```python
from build123d import *

# Parameters (mm, degrees)
F1_DEPTH = 2.794
F2_R     = 23.5
F3_DEPTH = 15
F5_D     = 12.1
F7_D     = 9
F7_DEPTH = 3
F7_TIP   = 2.7038727856
F9_D     = 17
F9_DEPTH = 2
F9_TIP   = 5.1073152617


with BuildPart() as f1:
    # F0 (on Front) → F1 (new body)
    with BuildSketch(Plane.XZ):
        Polygon((-22.3028203132, 16.203947452), (-27.5678019971, 0), (-22.3028203132, -16.203947452), (-8.5189193147, -26.2185377292), (8.5189193147, -26.2185377292), (22.3028203132, -16.203947452), (27.5678019971, 0), (22.3028203132, 16.203947452), (8.5189193147, 26.2185377292), (-8.5189193147, 26.2185377292), align=None)
    extrude(amount=F1_DEPTH)

    # F2 (on face) → F3 (join)
    with BuildSketch(Plane.XZ.offset(2.794)):
        Circle(F2_R)
    extrude(amount=F3_DEPTH)

    # F5 (through all)
    with Locations(Plane.XZ.offset(17.794)):
        with Locations((-14, 0), (0, 14), (14, 0), (0, -14)):
            Hole(F5_D / 2)

    # F7
    with Locations(Plane(origin=(0, 0, 0), x_dir=(-1, 0, 0), z_dir=(0, 1, 0))):
        with Locations((0, 0)):
            Hole(F7_D / 2, depth=F7_DEPTH)
            with Locations((0, 0, -(F7_DEPTH + F7_TIP / 2))):  # 118° drill point
                Cone(0, F7_D / 2, F7_TIP, mode=Mode.SUBTRACT)

    # F9
    with Locations(Plane(origin=(0, 0, 0), x_dir=(-1, 0, 0), z_dir=(0, 1, 0))):
        with Locations((-14, 0), (0, 14), (14, 0), (0, -14)):
            Hole(F9_D / 2, depth=F9_DEPTH)
            with Locations((0, 0, -(F9_DEPTH + F9_TIP / 2))):  # 118° drill point
                Cone(0, F9_D / 2, F9_TIP, mode=Mode.SUBTRACT)


solid = f1.part
```
Design review of the part built by this model. Coordinates are the model's own, in mm. A direction names the side the tool comes from. Coordinates: 2 decimals unless noted, no trailing zeros. Loops run counter-clockwise (first coordinate to the right, second up) from the corner with the lowest first, then second, coordinate; pieces in that order, holes last.
Q1. Tool access review of faces 4 (the face through (-0.59, -1.52, 4.46)), 5 (the face through (22.4, -10.2, 7.1)), 6 (the face through (8.411, -10.533, -2.317)): name each direction out of +Z, -Z, +X, -X, +Y, -Y from which nothing blocks a thin tool from reaching the whole face with its end or side.
Reported:
face 4: +Y
face 5: -Y
face 6: +Y, -Y
Q2. We need section A-A on x = -14. State the section outline as (y, z) points.
Reported:
outline: (-17.79, -18.87) - (-2.79, -18.87) - (-2.79, -22.24) - (0, -22.24) - (0, -8.5) - (-2, -8.5) - (-3.47, -6.05) - (-17.79, -6.05) - close; (-17.79, 6.05) - (-3.47, 6.05) - (-2, 8.5) - (0, 8.5) - (0, 22.24) - (-2.79, 22.24) - (-2.79, 18.87) - (-17.79, 18.87) - close
Q3. For pin 1 (1.5 mm diameter, centred on y = -9.5, z = 5, fed in from +X); pin 2 (10 mm diameter, centred on x = 16, z = -1, fed in from +Y); pin 3 (12 mm diameter, centred on x = -9, z = 3, fed in from +Y); pin 4 (5 mm diameter, centred on x = -2.5, y = -13.5, fed in from +Z), all flat-tipped, find the tip position at first contact; note any pin that passes through.
Reported:
pin 1: stops at x = 23.11
pin 2: stops at y = -2.76
pin 3: stops at y = 0
pin 4: stops at z = 23.5
Q4. We need section D-D on z = 3. State how many separate pieces and enclosed holes the cut face has, and give its area (3 significant figures).
Reported:
separate pieces: 3
enclosed holes: 0
area: 420 mm2
Q5. The part is to be moulded in two halves that separate along Z. For faces 1 (the face through (-19.92, -3.38, 1.86)), 2 (the face through (0, -1, 26.219)), 3 (the face through (-15.51, -1.38, -21.14)), say which applies: +Z half, -Z half, draft (parallel to the pull), parting line (faces both ways), or undercut.
Reported:
face 1: undercut
face 2: +Z half
face 3: -Z half
Q6. We need section B-B on z = 14. State the section outline as (x, y) points.
Reported:
outline: (-23.02, -2.79) - (-18.87, -2.79) - (-18.87, -17.79) - (-6.05, -17.79) - (-6.05, -3.47) - (-8.5, -2) - (-8.5, 0) - (-23.02, 0) - close; (6.05, -17.79) - (18.87, -17.79) - (18.87, -2.79) - (23.02, -2.79) - (23.02, 0) - (8.5, 0) - (8.5, -2) - (6.05, -3.47) - close
Q7. We need section C-C on y = -7. State the section outline as (x, z) points, and give its area (3 significant figures).
Reported:
outline: circle Ø47 at (0, 0); hole circle Ø12.1 at (-14, 0); hole circle Ø12.1 at (0, -14); hole circle Ø12.1 at (0, 14); hole circle Ø12.1 at (14, 0)
area: 1,270 mm2
Q8. To check wall thickness, follow line 1 (Z direction, x = 0, y = -1.4); line 2 (Z direction, x = 0, y = -13); line 3 (X direction, y = -1.4, z = 0). State the ranges of each line that lie inside material, in increasing order.
Reported:
line 1: z = -26.22 to -22.5, -5.5 to -4.5, 4.5 to 5.5, 22.5 to 26.22
line 2: z = -23.5 to -20.05, -7.95 to 7.95, 20.05 to 23.5
line 3: x = -27.57 to -22.5, -5.5 to -4.5, 4.5 to 5.5, 22.5 to 27.57
